Design review of the part built by this model. Coordinates are the model's own, in mm. A direction names the side the tool comes from. Give positions to 0.01 mm unless a question says otherwise; leave off trailing zeros. One line per item, written item: value. Start each with the question number.
1) Wall thickness on line 1 along Y through (x, z) = (35, 2.75); line 2 along Y through (x, z) = (0, 2.2); line 3 along Y through (x, z) = (43, 1.8): over which ranges is each line inside the solid? List them lowest first. Write a range as from..to.
2) Tool access review of faces 1 (the face through (23, 26, 0)), 2 (the face through (-35.05, 28.62, 1.97)): name each direction out of +Z, -Z, +X, -X, +Y, -Y from which nothing blocks a thin tool from reaching the whole face with its end or side.
3) For pin 1 (1.5 mm diameter, centred on x = 19, z = 0.5, fed in from +Y); pin 2 (6 mm diameter, centred on x = -28.5, y = -25.5, fed in from +Z), all flat-tipped, find the tip position at first contact; note any pin that passes through.
4) The part is to be moulded in two halves that separate along X. For faces 3 (the face through (3.97, 67.75, 3.91)), 4 (the face through (51.303, 45.78, 0.09)), 5 (the face through (23, 26, 4)), 6 (the face through (28.62, 35.05, 1.97)), say which applies: released by +X, released by -X, zero draft, split by the parting line, or undercut.
5) Consider section A-A (x = 3.5). State how many separate pieces and enclosed holes the cut face has, plus the area to 3 significant figures.
from build123d import *

# Parameters (mm, degrees)
SKETCH1_R           = 32.5
BOSS_EXTRUDE1_DEPTH = 4
FILLET1_R           = 0.3


with BuildPart() as part:
    # Sketch1 → Boss-Extrude1 (new body)
    with BuildSketch(Plane.XY):
        with BuildLine():
            Line((40.513754338, 97.768275578), (-31.667544375, 38.693237565))
            ThreePointArc((-31.667544375, 38.693237565), (-22.079944387, -44.860629241), (49.977742159, -1.491740146))
            Line((49.977742159, -1.491740146), (52.760547318, 91.740528921))
            ThreePointArc((52.760547318, 91.740528921), (48.575877652, 98.693384329), (40.513754338, 97.768275578))
        make_face()
        with BuildLine():
            Line((44.429740051, 82.343780573), (40.013751174, 73.371654725))
            ThreePointArc((40.013751174, 73.371654725), (35.32791102, 71.777006785), (33.73326308, 76.462846939))
            Line((33.73326308, 76.462846939), (38.149251957, 85.434972787))
            ThreePointArc((38.149251957, 85.434972787), (42.835092111, 87.029620727), (44.429740051, 82.343780573))
        make_face(mode=Mode.SUBTRACT)
        with BuildLine():
            ThreePointArc((27.168436627, 25.484084273), (23.609666403, 28.812256981), (19.646928241, 31.647443984))
            ThreePointArc((19.646928241, 31.647443984), (18.358282255, 37.155564491), (23.866402763, 38.444210477))
            ThreePointArc((23.866402763, 38.444210477), (28.680198785, 35.000124252), (33.003268654, 30.957176198))
            ThreePointArc((33.003268654, 30.957176198), (32.822398603, 25.303214222), (27.168436627, 25.484084273))
        make_face(mode=Mode.SUBTRACT)
        with BuildLine():
            ThreePointArc((-23.866402763, -38.444210477), (-28.680198785, -35.000124252), (-33.003268654, -30.957176198))
            ThreePointArc((-33.003268654, -30.957176198), (-32.822398603, -25.303214222), (-27.168436627, -25.484084273))
            ThreePointArc((-27.168436627, -25.484084273), (-23.609666403, -28.812256981), (-19.646928241, -31.647443984))
            ThreePointArc((-19.646928241, -31.647443984), (-18.358282255, -37.155564491), (-23.866402763, -38.444210477))
        make_face(mode=Mode.SUBTRACT)
        with BuildLine():
            ThreePointArc((-44.060257161, -10.30806669), (-45.028788248, -4.468862155), (-45.226864283, 1.446805851))
            ThreePointArc((-45.226864283, 1.446805851), (-41.101014989, 5.316866265), (-37.230954575, 1.191016971))
            ThreePointArc((-37.230954575, 1.191016971), (-37.067897508, -3.678787077), (-36.270598437, -8.485646059))
            ThreePointArc((-36.270598437, -8.485646059), (-39.254217484, -13.291685737), (-44.060257161, -10.30806669))
        make_face(mode=Mode.SUBTRACT)
        Circle(SKETCH1_R, mode=Mode.SUBTRACT)
        with BuildLine():
            ThreePointArc((10.30806669, -44.060257161), (4.468862155, -45.028788248), (-1.446805851, -45.226864283))
            ThreePointArc((-1.446805851, -45.226864283), (-5.316866265, -41.101014989), (-1.191016971, -37.230954575))
            ThreePointArc((-1.191016971, -37.230954575), (3.678787077, -37.067897508), (8.485646059, -36.270598437))
            ThreePointArc((8.485646059, -36.270598437), (13.291685737, -39.254217484), (10.30806669, -44.060257161))
        make_face(mode=Mode.SUBTRACT)
        with BuildLine():
            ThreePointArc((38.444210477, -23.866402763), (35.000124252, -28.680198785), (30.957176198, -33.003268654))
            ThreePointArc((30.957176198, -33.003268654), (25.303214222, -32.822398603), (25.484084273, -27.168436627))
            ThreePointArc((25.484084273, -27.168436627), (28.812256981, -23.609666403), (31.647443984, -19.646928241))
            ThreePointArc((31.647443984, -19.646928241), (37.155564491, -18.358282255), (38.444210477, -23.866402763))
        make_face(mode=Mode.SUBTRACT)
        with BuildLine():
            ThreePointArc((44.060257161, 10.30806669), (45.028788248, 4.468862155), (45.226864283, -1.446805851))
            ThreePointArc((45.226864283, -1.446805851), (41.101014989, -5.316866265), (37.230954575, -1.191016971))
            ThreePointArc((37.230954575, -1.191016971), (37.067897508, 3.678787077), (36.270598437, 8.485646059))
            ThreePointArc((36.270598437, 8.485646059), (39.254217484, 13.291685737), (44.060257161, 10.30806669))
        make_face(mode=Mode.SUBTRACT)
        with BuildLine():
            ThreePointArc((-38.444210477, 23.866402763), (-35.000124252, 28.680198785), (-30.957176198, 33.003268654))
            ThreePointArc((-30.957176198, 33.003268654), (-25.303214222, 32.822398603), (-25.484084273, 27.168436627))
            ThreePointArc((-25.484084273, 27.168436627), (-28.812256981, 23.609666403), (-31.647443984, 19.646928241))
            ThreePointArc((-31.647443984, 19.646928241), (-37.155564491, 18.358282255), (-38.444210477, 23.866402763))
        make_face(mode=Mode.SUBTRACT)
        with BuildLine():
            ThreePointArc((-10.30806669, 44.060257161), (-4.468862155, 45.028788248), (1.446805851, 45.226864283))
            ThreePointArc((1.446805851, 45.226864283), (5.316866265, 41.101014989), (1.191016971, 37.230954575))
            ThreePointArc((1.191016971, 37.230954575), (-3.678787077, 37.067897508), (-8.485646059, 36.270598437))
            ThreePointArc((-8.485646059, 36.270598437), (-13.291685737, 39.254217484), (-10.30806669, 44.060257161))
        make_face(mode=Mode.SUBTRACT)
    extrude(amount=BOSS_EXTRUDE1_DEPTH)

    # Fillet1
    fillet1_edges = [part.edges().sort_by_distance(p)[0] for p in [
        (-32.5, 0, 4),
        (48.575877652, 98.693384329, 4),
        (4.423104981, 68.230756572, 4),
        (-22.079944387, -44.860629241, 4),
        (51.369144738, 45.124394387, 4),
        (-32.5, 0, 0),
        (51.369144738, 45.124394387, 0),
        (-22.079944387, -44.860629241, 0),
        (4.423104981, 68.230756572, 0),
        (48.575877652, 98.693384329, 0),
    ]]
    fillet(fillet1_edges, radius=FILLET1_R)


solid = part.part
Checked values:
1. line 1: y = -35.71..-28.68, -17.76..71.96, 79.04..93.26
1. line 2: y = -50..-45.25, -37.25..-32.5, 32.5..37.25, 45.25..64.61
1. line 3: y = -25.51..-4.91, 12.22..79.44, 86.94..99.11
2. face 1: -Z, +X, -X, +Y, -Y
2. face 2: +Z, -Z
3. pin 1: stops at y = 80.77
3. pin 2: stops at z = 4
4. face 3: released by -X
4. face 4: released by +X
4. face 5: zero draft
4. face 6: undercut
5. separate pieces: 4
5. enclosed holes: 0
5. area: 152 mm^2
